Check sheet for the drawn part. Datum: minimum x, y, z corner. Units: mm. Give positions to 0.01 mm unless a question says otherwise; leave off trailing zeros. Order: outer loops, then holes, each group sorted by start corner. A loop starts at its lowest first (then second) coordinate and runs counter-clockwise, first axis right, second up.
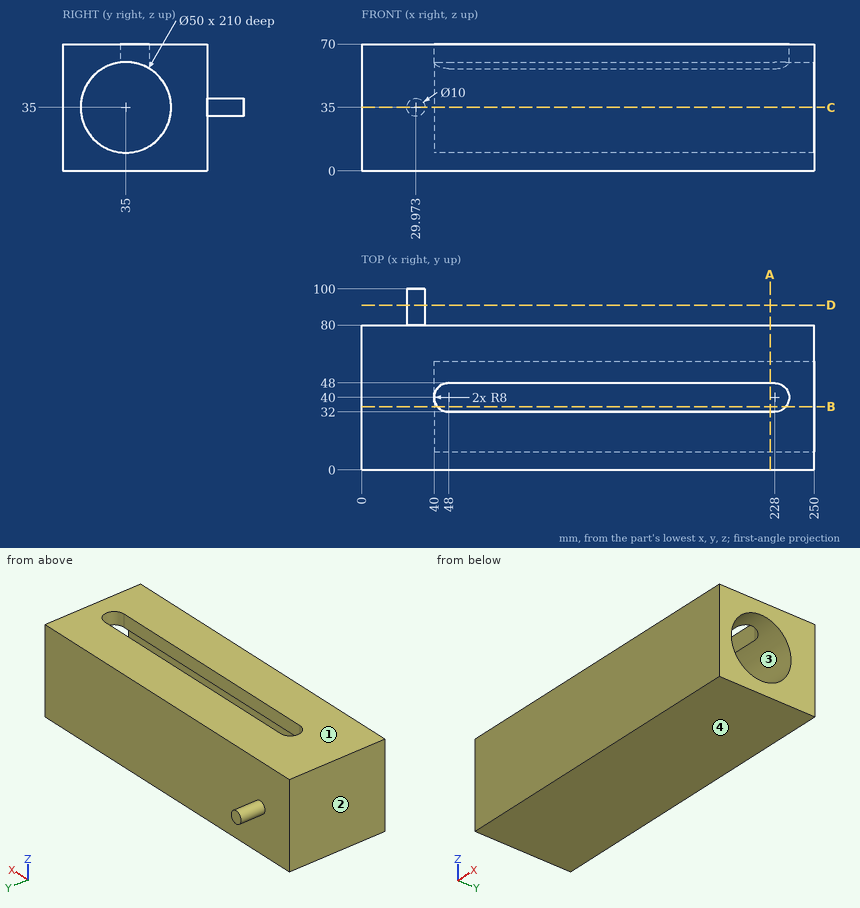
Item 1: Sectioned sample at D-D (y = 91). Enter the section's corners in (x, z).
Reported:
outline: circle Ø10 at (29.97, 35)
Item 2: Sectioned sample at C-C (z = 35). Enter the section's corners in (x, y), and give its area (3 significant figures).
Reported:
outline: (0, 0) - (250, 0) - (250, 10) - (40, 10) - (40, 60) - (250, 60) - (250, 80) - (34.97, 80) - (34.97, 100) - (24.97, 100) - (24.97, 80) - (0, 80) - close
area: 9,700 mm2
Item 3: Sectioned sample at B-B (y = 35). Enter the section's corners in (x, z) (3 decimals), and give its area (3 significant figures).
Reported:
outline: (0, 0) - (250, 0) - (250, 10) - (40, 10) - (40, 60) - (41.755, 60) - (41.755, 70) - (0, 70) - close; (234.245, 60) - (250, 60) - (250, 70) - (234.245, 70) - close
area: 5,080 mm2
Item 4: Scan lines: L1, parallel to Y at x = 83, z = 35; L2, parallel to Z at x = 206, y = 35; L3, parallel to Y at x = 63, z = 15. Record each from-to range of solid material in increasing order.
Reported:
L1: y = 0 to 10, 60 to 80
L2: z = 0 to 10
L3: y = 0 to 20, 50 to 80
Item 5: Draft check along Z on the marked faces 1, 2, 3 and 4. Enter one of: released by +Z, released by -Z, zero draft, split by the parting line, or undercut.
Reported:
face 1: released by +Z
face 2: zero draft
face 3: undercut
face 4: released by -Z
Item 6: Gauge pin test, flat ends, axial feed: pin 1 (21 mm diameter, centred on x = 87, z = 45.5, fed in from +Y); pin 2 (12 mm diameter, centred on y = 86.5, z = 20, fed in from +X); pin 3 (10 mm diameter, centred on y = 41.5, z = 52.5, fed in from +X). Record the tip position at first contact, or that the pin passes through.
Reported:
pin 1: stops at y = 80
pin 2: passes through
pin 3: stops at x = 40
Item 7: Sectioned sample at A-A (x = 225.5). Enter the section's corners in (y, z).
Reported:
outline: (0, 0) - (80, 0) - (80, 70) - (48, 70) - (48, 56.35) arc R25 cw (long way) to (32, 59.82) - (32, 70) - (0, 70) - close
